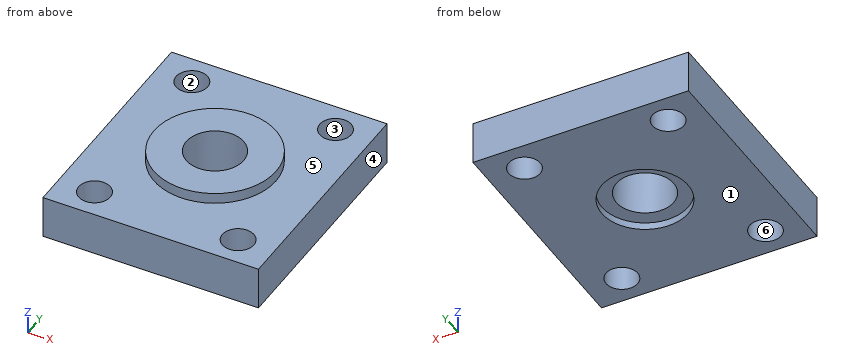
```python
from build123d import *

# Parameters (mm, degrees)
F0_W     = 30
F0_H     = 33
F0_R     = 4
F1_DEPTH = 6
F2_R     = 8.5
F2_R_2   = 4
F3_DEPTH = 1.5
F4_R     = 6
F4_R_2   = 4
F5_DEPTH = 1
F7_D     = 4.4


with BuildPart() as f1:
    # F0 (on Top) → F1 (new body)
    with BuildSketch(Plane.XY):
        Rectangle(F0_W, F0_H)
        Circle(F0_R, mode=Mode.SUBTRACT)
    extrude(amount=F1_DEPTH)

    # F2 (on face) → F3 (join)
    with BuildSketch(Plane.XY.offset(6)):
        Circle(F2_R)
        Circle(F2_R_2, mode=Mode.SUBTRACT)
    extrude(amount=F3_DEPTH)

    # F4 (on face) → F5 (cut)
    with BuildSketch(Plane(origin=(0, 0, 0), x_dir=(1, 0, 0), z_dir=(0, 0, -1))):
        Circle(F4_R)
        Circle(F4_R_2, mode=Mode.SUBTRACT)
    extrude(amount=-F5_DEPTH, mode=Mode.SUBTRACT)

    # F7 (through all)
    with Locations(Plane.XY.offset(6)):
        with Locations((-10, 12.5), (10, 12.5), (10, -12.5), (-10, -12.5)):
            Hole(F7_D / 2)


solid = f1.part
```
Check sheet for the modelled part. Datum: model origin and axes. Units: mm. Face numbers are marked on the shaded views. A direction names the side the tool comes from. Coordinates: 2 decimals unless noted, no trailing zeros. Order: outer loops, then holes, each group sorted by start corner. A loop starts at its lowest first (then second) coordinate and runs counter-clockwise, first axis right, second up. Notation, with made-up numbers: M 66.5,0 L 90.5,0 A17 ccw 90.5,14 Z; hole C 89,65.25 d11. An arc over 180 degrees is marked long. Write each question's results on one line, items separated by ' | '. Start each with the question number.
1. Cross-section at D-D on x = -2.5. Record the cut outline in (y, z), and give its area (3 significant figures).
2. Mould release check, pull along X, two halves, no side actions. Record for the marked faces 1, 2, 3 and 4: +X half, -X half, draft (parallel to the pull), parting line (faces both ways), or undercut.
3. Access from +Z, -Z, +X, -X, +Y, -Y to the whole of each face (thin tool, end or side, straight path). Record for the marked faces 5 and 6.
4. Material ranges on probe 1 along Y at (x, z) = (-10, 2.95); probe 2 along X at (y, z) = (0, 0.85); probe 3 along X at (y, z) = (-11, 1), recorded low to high.
5. Cross-section at A-A on y = -12.5. Record the cut outline in (x, z), and give its area (3 significant figures).
6. Cross-section at B-B on x = 10. Record the cut outline in (y, z), and give its area (3 significant figures).
7. Go/stop test with a flat-tipped pin: P1, Ø7, axis at x = 10, y = -12.5, coming from the +Z side. Record where the tip stops, or that it passes through.
8. Cross-section at C-C on z = 5.25. Record the cut outline in (x, y).
Checks:
1) outline: M -16.5,0 L -5.45,0 L -5.45,1 L -3.12,1 L -3.12,7.5 L -8.12,7.5 L -8.12,6 L -16.5,6 Z; M 3.12,1 L 5.45,1 L 5.45,0 L 16.5,0 L 16.5,6 L 8.12,6 L 8.12,7.5 L 3.12,7.5 Z | area: 171 mm²
2) face 1: draft | face 2: undercut | face 3: undercut | face 4: +X half
3) face 5: +Z | face 6: +Z, -Z
4) probe 1: y = -16.5 to -14.7, -10.3 to 10.3, 14.7 to 16.5 | probe 2: x = -15 to -6, 6 to 15 | probe 3: x = -15 to -11.61, -8.39 to 8.39, 11.61 to 15
5) outline: M -15,0 L -12.2,0 L -12.2,6 L -15,6 Z; M -7.8,0 L 7.8,0 L 7.8,6 L -7.8,6 Z; M 12.2,0 L 15,0 L 15,6 L 12.2,6 Z | area: 127 mm²
6) outline: M -16.5,0 L -14.7,0 L -14.7,6 L -16.5,6 Z; M -10.3,0 L 10.3,0 L 10.3,6 L -10.3,6 Z; M 14.7,0 L 16.5,0 L 16.5,6 L 14.7,6 Z | area: 145 mm²
7) P1: stops at z = 6
8) outline: M -15,-16.5 L 15,-16.5 L 15,16.5 L -15,16.5 Z; hole C -10,-12.5 d4.4; hole C -10,12.5 d4.4; hole C 0,0 d8; hole C 10,-12.5 d4.4; hole C 10,12.5 d4.4
